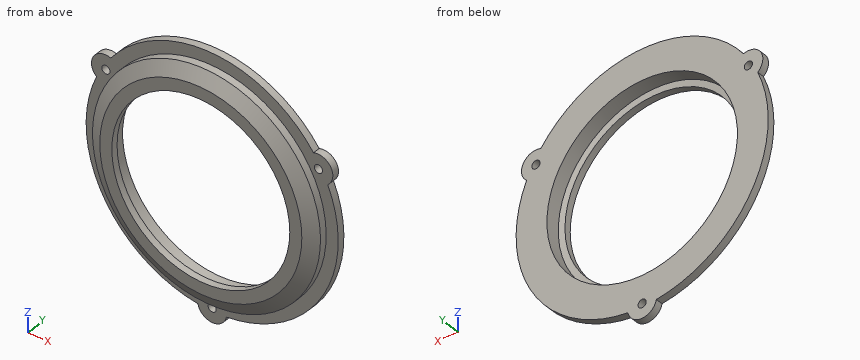
from build123d import *

# Parameters (mm, degrees)
BOSS_EXTRU_2_DEPTH           = 3
D_GAGEMENT_M32_D             = 3.4
R_P_TITION_CIRCULAIRE1_COUNT = 3


with BuildPart() as part:
    # Esquisse1 → Révolution1 (revolve)
    with BuildSketch(Plane.XY, mode=Mode.PRIVATE) as r_volution1_sk:
        with BuildLine():
            Line((-39.6, 5.132876041), (-39.6, -0.867123959))
            ThreePointArc((-39.6, -0.867123959), (-38.300433177, -0.984457181), (-37, -1.091763109))
            Line((-37, -1.091763109), (-37, -3.867123959))
            Line((-37, -3.867123959), (-42, -3.867123959))
            Line((-42, -3.867123959), (-47.4, -0.867123959))
            Line((-47.4, -0.867123959), (-47.4, 2.132876041))
            Line((-47.4, 2.132876041), (-52.4, 2.132876041))
            Line((-52.4, 2.132876041), (-52.4, 5.132876041))
            Line((-52.4, 5.132876041), (-39.6, 5.132876041))
        make_face()
    revolve(r_volution1_sk.sketch.rotate(Axis((0, 0, 0), (0, 1, 0)), 270), axis=Axis((0, 0, 0), (0, 1, 0)))

    # Esquisse2 → Boss.-Extru.2 (add)
    with BuildSketch(Plane(origin=(0, 5.132876041, 0), x_dir=(1, 0, 0), z_dir=(0, 1, 0))):
        with BuildLine():
            Line((-5.904494785, 52.06627451), (0, 51))
            Line((0, 51), (5.904494785, 52.06627451))
            ThreePointArc((5.904494785, 52.06627451), (0, 57), (-5.904494785, 52.06627451))
        make_face()
    boss_extru_2 = extrude(amount=-BOSS_EXTRU_2_DEPTH)

    # Dégagement M32 (through all)
    with Locations(Plane(origin=(0, 5.132876041, 0), x_dir=(1, 0, 0), z_dir=(0, 1, 0))):
        with Locations((0, 51)):
            d_gagement_m32 = Hole(D_GAGEMENT_M32_D / 2)

    # Répétition circulaire1: Boss.-Extru.2, Dégagement M32 ×3 about axis
    r_p_tition_circulaire1_axis = Axis((0, 0, 0), (0, 1, 0))
    add([boss_extru_2.rotate(r_p_tition_circulaire1_axis, i * 360 / R_P_TITION_CIRCULAIRE1_COUNT) for i in range(1, R_P_TITION_CIRCULAIRE1_COUNT)])
    add([d_gagement_m32.rotate(r_p_tition_circulaire1_axis, i * 360 / R_P_TITION_CIRCULAIRE1_COUNT) for i in range(1, R_P_TITION_CIRCULAIRE1_COUNT)], mode=Mode.SUBTRACT)


solid = part.part
Input: part model. Units: mm. Frame: model coordinates. Coordinates: 2 decimals unless noted, no trailing zeros.
1. Cut plane A-A, the plane z = 25.5. Count the separate pieces of the cut face and the enclosed holes in it, plus the area to 3 significant figures.
Checked values:
separate pieces: 4
enclosed holes: 0
area: 215 mm2
2. Contact query for flat-ended pins moving along their axis: P1, Ø4, axis at x = -8.5, y = 4, coming from the -Z side; P2, Ø4.5, axis at x = 44.17, z = 25.5, coming from the +Y side; P3, Ø3, axis at x = -3.5, y = 0, coming from the -Z side; P4, Ø4, axis at x = -5, y = -2, coming from the -Z side. Output: stop coordinate, or through.
Checked values:
P1: stops at z = -52
P2: stops at y = 5.13
P3: stops at z = -47.36
P4: stops at z = -47.28
3. Ray query, line 1 along Y through (x, z) = (-47, 17.5); line 2 along X through (y, z) = (-0.75, -28.5); line 3 along Z through (x, y) = (27.5, 2.25). Return the intervals inside material, ascending.
Checked values:
line 1: y = 2.13 to 5.13
line 2: x = -37.87 to -27.49, 27.49 to 37.87
line 3: z = -44.6 to -28.49, 28.49 to 44.6
